```python
from build123d import *

# Parameters (mm, degrees)
SKETCH_1_R      = 3.5
SKETCH_1_R_2    = 2.5
EXTRUDE_1_DEPTH = 5
EXTRUDE_START   = -3
SKETCH_2_R      = 0.625
SKETCH_2_R_2    = 1.625
SKETCH_2_R_3    = 2.5
SKETCH_2_R_4    = 1.5
EXTRUDE_2_DEPTH = 2
EXTRUDE_3_DEPTH = 1
CHAMFER_1_SIZE  = 1


with BuildPart() as part:
    # Эскиз1 → Бобышка-Вытянуть1 (new body)
    with BuildSketch(Plane.XY):
        Circle(SKETCH_1_R)
        Circle(SKETCH_1_R_2, mode=Mode.SUBTRACT)
    extrude(amount=EXTRUDE_1_DEPTH)

    # Эскиз2 → Бобышка-Вытянуть2 (add)
    # profile 1 of 5: a face of its own
    with BuildSketch(Plane.XY.offset(5).offset(EXTRUDE_START)):
        with BuildLine():
            Line((-0.809199831, 3.405171895), (-16, 1.625))
            ThreePointArc((-16, 1.625), (-14.850951481, 1.149048519), (-14.375, 0))
            ThreePointArc((-14.375, 0), (-14.850951481, -1.149048519), (-16, -1.625))
            Line((-16, -1.625), (-0.809199831, -3.405171895))
            ThreePointArc((-0.809199831, -3.405171895), (-3.5, 0), (-0.809199831, 3.405171895))
        make_face()
        with Locations((-13.37, 0)):
            Circle(SKETCH_2_R, mode=Mode.SUBTRACT)
        with Locations((-10.74, 0)):
            Circle(SKETCH_2_R, mode=Mode.SUBTRACT)
        with Locations((-8.11, 0)):
            Circle(SKETCH_2_R, mode=Mode.SUBTRACT)
        with Locations((-5.48, 0)):
            Circle(SKETCH_2_R, mode=Mode.SUBTRACT)
    # profile 2 of 5: a face of its own
    with BuildSketch(Plane.XY.offset(5).offset(EXTRUDE_START)):
        with Locations((-16, 0)):
            Circle(SKETCH_2_R_2)
        with Locations((-16, 0)):
            Circle(SKETCH_2_R, mode=Mode.SUBTRACT)
    # profile 3 of 5: a face of its own
    with BuildSketch(Plane.XY.offset(5).offset(EXTRUDE_START)):
        with BuildLine():
            Line((16, 1.625), (0.809199831, 3.405171895))
            ThreePointArc((0.809199831, 3.405171895), (2.746106281, 2.170000068), (3.5, 0))
            ThreePointArc((3.5, 0), (2.746106281, -2.170000068), (0.809199831, -3.405171895))
            Line((0.809199831, -3.405171895), (16, -1.625))
            ThreePointArc((16, -1.625), (14.375, 0), (16, 1.625))
        make_face()
        with Locations((5.48, 0)):
            Circle(SKETCH_2_R, mode=Mode.SUBTRACT)
        with Locations((8.11, 0)):
            Circle(SKETCH_2_R, mode=Mode.SUBTRACT)
        with Locations((10.74, 0)):
            Circle(SKETCH_2_R, mode=Mode.SUBTRACT)
        with Locations((13.37, 0)):
            Circle(SKETCH_2_R, mode=Mode.SUBTRACT)
    # profile 4 of 5: a face of its own
    with BuildSketch(Plane.XY.offset(5).offset(EXTRUDE_START)):
        with Locations((16, 0)):
            Circle(SKETCH_2_R_2)
        with Locations((16, 0)):
            Circle(SKETCH_2_R, mode=Mode.SUBTRACT)
    # profile 5 of 5: a face of its own
    with BuildSketch(Plane.XY.offset(5).offset(EXTRUDE_START)):
        Circle(SKETCH_2_R_3)
        Circle(SKETCH_2_R_4, mode=Mode.SUBTRACT)
    extrude(amount=EXTRUDE_2_DEPTH)

    # Эскиз3 → Бобышка-Вытянуть3 (add)
    with BuildSketch(Plane.XY.offset(4)):
        with BuildLine():
            ThreePointArc((-2.511691412, 2.4375), (-1.729501919, 3.04283143), (-0.809199831, 3.405171895))
            Line((-0.809199831, 3.405171895), (-4.8, 2.9375))
            Line((-4.8, 2.9375), (-4.8, 2.4375))
            Line((-4.8, 2.4375), (-2.511691412, 2.4375))
        make_face()
        with BuildLine():
            ThreePointArc((-3.491060011, -0.25), (-3.5, 0), (-3.491060011, 0.25))
            Line((-3.491060011, 0.25), (-4.8, 0.25))
            Line((-4.8, 0.25), (-4.8, -0.25))
            Line((-4.8, -0.25), (-3.491060011, -0.25))
        make_face()
        with BuildLine():
            ThreePointArc((-0.809199831, -3.405171895), (-1.729501919, -3.04283143), (-2.511691412, -2.4375))
            Line((-2.511691412, -2.4375), (-4.8, -2.4375))
            Line((-4.8, -2.4375), (-4.8, -2.9375))
            Line((-4.8, -2.9375), (-0.809199831, -3.405171895))
        make_face()
        with BuildLine():
            Line((4.8, -2.4375), (2.511691412, -2.4375))
            ThreePointArc((2.511691412, -2.4375), (1.729501919, -3.04283143), (0.809199831, -3.405171895))
            Line((0.809199831, -3.405171895), (4.8, -2.9375))
            Line((4.8, -2.9375), (4.8, -2.4375))
        make_face()
        with BuildLine():
            Line((4.8, 0.25), (3.491060011, 0.25))
            ThreePointArc((3.491060011, 0.25), (3.497764289, 0.125079898), (3.5, 0))
            ThreePointArc((3.5, 0), (3.497764289, -0.125079898), (3.491060011, -0.25))
            Line((3.491060011, -0.25), (4.8, -0.25))
            Line((4.8, -0.25), (4.8, 0.25))
        make_face()
        with BuildLine():
            Line((4.8, 2.9375), (0.809199831, 3.405171895))
            ThreePointArc((0.809199831, 3.405171895), (1.729501919, 3.04283143), (2.511691412, 2.4375))
            Line((2.511691412, 2.4375), (4.8, 2.4375))
            Line((4.8, 2.4375), (4.8, 2.9375))
        make_face()
    extrude(amount=EXTRUDE_3_DEPTH)

    # Фаска1
    chamfer_1_edges = [part.edges().sort_by_distance(p)[0] for p in [
        (4.8, 2.6875, 5),
        (4.8, 0, 5),
        (4.8, -2.6875, 5),
        (-4.8, -2.6875, 5),
        (-4.8, 0, 5),
        (-4.8, 2.6875, 5),
    ]]
    chamfer(chamfer_1_edges, length=CHAMFER_1_SIZE - 0.0001)  # a hair under: the kernel refuses the full size


solid = part.part
```
The model under review builds one solid part; all positions refer to its coordinate system, in mm. A direction names the side the tool comes from. Round coordinates to 2 decimals unless told otherwise and drop trailing zeros. Order: outer loops, then holes, each group sorted by start corner. A loop starts at its lowest first (then second) coordinate and runs counter-clockwise, first axis right, second up.
Item 1: Draft analysis for pull direction Y (two halves, no side actions). For faces 1 (the cylindrical face through (-15.423, -0.239, 2.986)), 2 (the flat face through (9, 0, 2)), 3 (the cylindrical face through (-17.625, 0.036, 2.986)), state which applies: released by +Y, released by -Y, zero draft, split by the parting line, or undercut.
Working result:
face 1: undercut
face 2: zero draft
face 3: split by the parting line
Item 2: For pin 1 (2 mm diameter, centred on x = 16, y = 0, fed in from +Z); pin 2 (2 mm diameter, centred on x = -12.5, y = 0.5, fed in from -Z); pin 3 (1.5 mm diameter, centred on x = -12.5, z = 4, fed in from -Y), all flat-tipped, find the tip position at first contact; note any pin that passes through.
Working result:
pin 1: stops at z = 4
pin 2: stops at z = 2
pin 3: stops at y = -2.12
Item 3: Add section D-D, the plane z = 1.25. State the section outline as (x, y) points.
Working result:
outline: circle Ø7 at (0, 0); hole circle Ø5 at (0, 0)
Item 4: Add section C-C, the plane y = -1. State the section outline as (x, z) points, and give its area (3 significant figures).
Working result:
outline: (-17.28, 2) - (-3.35, 2) - (-3.35, 0) - (-2.29, 0) - (-2.29, 2) - (-1.12, 2) - (-1.12, 4) - (-2.29, 4) - (-2.29, 5) - (-3.35, 5) - (-3.35, 4) - (-17.28, 4) - close; (1.12, 2) - (2.29, 2) - (2.29, 0) - (3.35, 0) - (3.35, 2) - (17.28, 2) - (17.28, 4) - (3.35, 4) - (3.35, 5) - (2.29, 5) - (2.29, 4) - (1.12, 4) - close
area: 71.0 mm2
Item 5: Add section B-B, the plane x = 0. State the section outline as (y, z) points.
Working result:
outline: (-3.5, 0) - (-2.5, 0) - (-2.5, 2) - (-1.5, 2) - (-1.5, 4) - (-2.5, 4) - (-2.5, 5) - (-3.5, 5) - close; (1.5, 2) - (2.5, 2) - (2.5, 0) - (3.5, 0) - (3.5, 5) - (2.5, 5) - (2.5, 4) - (1.5, 4) - close
Item 6: Machinability: for faces 4 (the cylindrical face through (-0.54, -2.44, 0.99)), 5 (the flat face through (4.3, 2.7, 4.5)), 6 (the flat face through (4, -0.25, 4.4)), which of the approach directions +Z, -Z, +X, -X, +Y, -Y give a long, thin tool a straight path to every point of the face, cutting with its end or side? Answer none if there is none.
Working result:
face 4: -Z
face 5: +Z, +X, +Y, -Y
face 6: +Z, +X
Item 7: Add section A-A, the plane z = 3.6. Count the separate pieces of the cut face and the enclosed holes in it, and give its area (3 significant figures).
Working result:
separate pieces: 1
enclosed holes: 11
area: 153 mm2
Item 8: To check wall thickness, follow probe 1 along Y at (x, z) = (0, 4.6); probe 2 along Y at (x, z) = (16, 2.65) (3 decimals); probe 3 along Z at (x, y) = (2.5, 2.5). State the ranges of each line that lie inside material, in increasing order.
Working result:
probe 1: y = -3.5 to -2.5, 2.5 to 3.5
probe 2: y = -1.625 to -0.625, 0.625 to 1.625
probe 3: z = 2 to 5
